from build123d import *

# Parameters (mm, degrees)
SKETCH1_W           = 25.4
SKETCH1_H           = 5
BOSS_EXTRUDE1_DEPTH = 5
SKETCH4_R           = 6.2
SKETCH4_R_2         = 5.2
BOSS_EXTRUDE2_DEPTH = 5
SKETCH5_R           = 5.2
CUT_EXTRUDE1_DEPTH  = 27.514083203


with BuildPart() as part:
    # Sketch1 → Boss-Extrude1 (new body)
    with BuildSketch(Plane(origin=(0, 0, 0), x_dir=(1, 0, 0), z_dir=(0, 1, 0))):
        with Locations((-11.05106383, 2.5)):
            Rectangle(SKETCH1_W, SKETCH1_H)
    extrude(amount=BOSS_EXTRUDE1_DEPTH)

    # Sketch4 → Boss-Extrude2 (add)
    with BuildSketch(Plane(origin=(0, 3.75, 2.165063509), x_dir=(1, 0, 0), z_dir=(0, 0.866025403784438, 0.500000000000001))):
        with Locations((-11.05106383, 2.5)):
            Circle(SKETCH4_R)
        with Locations((-11.05106383, 2.5)):
            Circle(SKETCH4_R_2, mode=Mode.SUBTRACT)
    extrude(amount=-BOSS_EXTRUDE2_DEPTH)

    # Sketch5 → Cut-Extrude1 (cut, through all)
    with BuildSketch(Plane(origin=(0, 3.75, 2.165063509), x_dir=(1, 0, 0), z_dir=(0, 0.866025403784438, 0.500000000000001))):
        with Locations(Location((-11.05106383, 2.5, 0), (0, 0, 270))):
            Circle(SKETCH5_R)
    extrude(amount=-CUT_EXTRUDE1_DEPTH, mode=Mode.SUBTRACT)


solid = part.part
Design review of the part built by this model. Coordinates are the model's own, in mm. Coordinates: 2 decimals unless noted, no trailing zeros. Order: outer loops, then holes, each group sorted by start corner. A loop starts at its lowest first (then second) coordinate and runs counter-clockwise, first axis right, second up. Notation, with made-up numbers: (88, 53.5) -> (101, 53.5) arc R20 ccw to (101, 69.5) -> close; hole circle Ø1 at (17, -32.75). An arc over 180 degrees is marked (long way). One line per item, written item: value.
1) We need section A-A, the plane x = -19.5. Give the boundary of the cut face in (y, z), then the cut area to 3 significant figures.
Output values:
outline: (0, -5) -> (5, -5) -> (5, 0) -> (0, 0) -> close
area: 25.0 mm2
2) Clearance check with flat-ended pins moving along their axes: P1, Ø4, axis at x = -2, z = -2.5, coming from the +Y side; P2, Ø1.5, axis at x = -21, y = 2.5, coming from the +Z side; P3, Ø4, axis at x = -3.5, z = -3, coming from the -Y side. State where each tip first meets the part, or that it passes through.
Output values:
P1: stops at y = 5
P2: stops at z = 0
P3: stops at y = 0
3) To check wall thickness, follow probe 1 along Y at (x, z) = (-22.5, -0.5); probe 2 along X at (y, z) = (2.5, 2); probe 3 along X at (y, z) = (3.25, 1.5). State the ranges of each line that lie inside material, in increasing order. Write a range as [from, to].
Output values:
probe 1: y = [0, 5]
probe 2: x = [-16.49, -15.31], [-6.79, -5.62]
probe 3: x = [-16.86, -15.77], [-6.33, -5.24]
4) Draft analysis for pull direction X (two halves, no side actions). For faces 1 (the face through (1.649, 2, -2)), 2 (the face through (-11.1, 3.5, -7.4)), 3 (the face through (-5.928, 2.296, -0.533)), state which applies: +X half, -X half, draft (parallel to the pull), parting line (faces both ways), or undercut.
Output values:
face 1: +X half
face 2: draft
face 3: undercut
